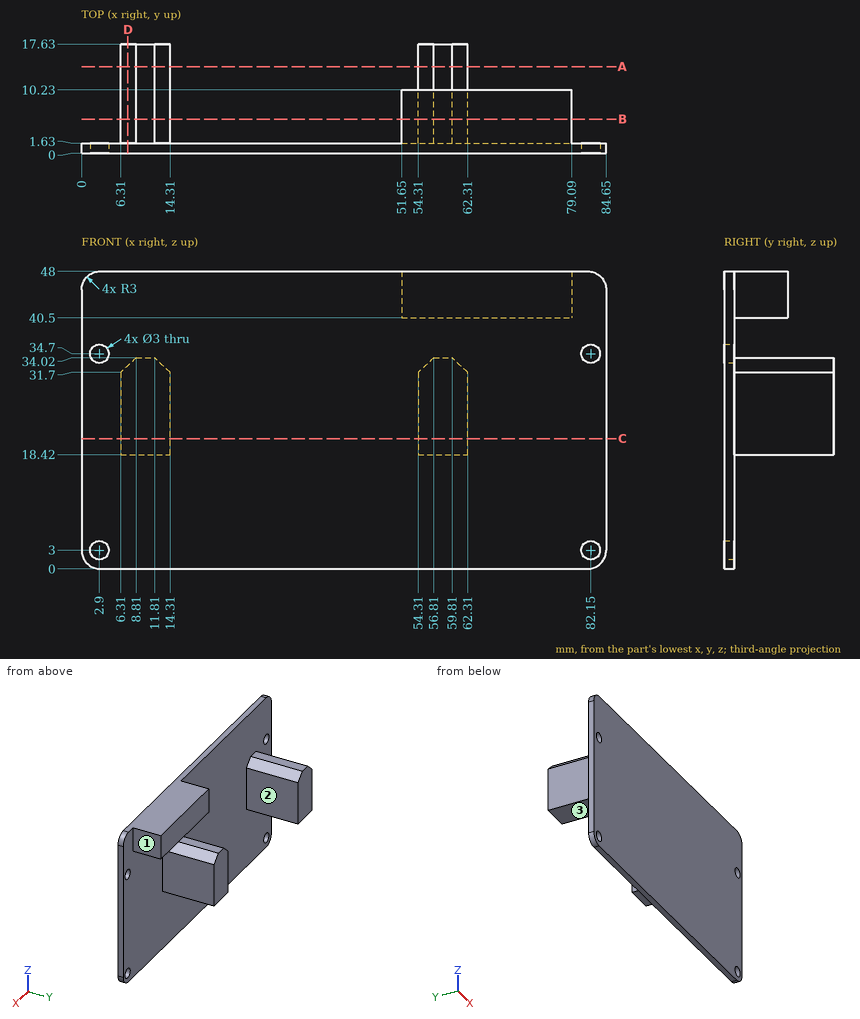
Here's the drawing with two shaded views (mm, measured from the low corner). I have some questions. A direction names the side the tool comes from. Give positions to 0.01 mm unless a question says otherwise; leave off trailing zeros. Loops run counter-clockwise (first coordinate to the right, second up) from the corner with the lowest first, then second, coordinate; pieces in that order, holes last. Notation, with made-up numbers: (-27, 18) -> (22, 18) arc R11 ccw to (22, 25) -> close; hole circle Ø5 at (0, -14). An arc over 180 degrees is marked (long way). Use one line per item in the form item = value.
1) If we section it at B-B (y = 5.5): Please give me the cut outline in (x, z), plus the area to 3 significant figures.
Answers:
outline = (6.31, 18.42) -> (14.31, 18.42) -> (14.31, 31.7) -> (11.81, 34.02) -> (8.81, 34.02) -> (6.31, 31.7) -> close; (51.65, 40.5) -> (79.09, 40.5) -> (79.09, 48) -> (51.65, 48) -> close; (54.31, 18.42) -> (62.31, 18.42) -> (62.31, 31.7) -> (59.81, 34.02) -> (56.81, 34.02) -> (54.31, 31.7) -> close
area = 444 mm²
2) I need wall thicknesses on line 1 along X through (y, z) = (1.3, 3); line 2 along Y through (x, z) = (15.5, 7); line 3 along Z through (x, y) = (11, 5.75). Which ranges of each line are inside material? Lowest first, please.
Answers:
line_1 = 0 to 1.4, 4.4 to 80.65, 83.65 to 84.65
line_2 = 0 to 1.63
line_3 = 18.42 to 34.02
3) If we section it at A-A (y = 14): Please give me the cut outline in (x, z).
Answers:
outline = (6.31, 18.42) -> (14.31, 18.42) -> (14.31, 31.7) -> (11.81, 34.02) -> (8.81, 34.02) -> (6.31, 31.7) -> close; (54.31, 18.42) -> (62.31, 18.42) -> (62.31, 31.7) -> (59.81, 34.02) -> (56.81, 34.02) -> (54.31, 31.7) -> close
4) For the marked faces 1, 2 and 3, which set-ups out of +Z, -Z, +X, -X, +Y, -Y let a thin tool reach every point of the face, with its end or its side?
Answers:
face_1 = +Z, -Z, +X, +Y
face_2 = +Z, -Z, +Y
face_3 = -Z, +X, -X, +Y
5) Will these pins go through, and if not, where does the flat tip stop? pin 1 (4 mm diameter, centred on x = 9, y = 11.5, fed in from -Z); pin 2 (9.5 mm diameter, centred on x = 68.5, y = 7.5, fed in from -Z); pin 3 (3 mm diameter, centred on x = 49.5, z = 12.5, fed in from +Y).
Answers:
pin_1 = 18.42
pin_2 = 40.5
pin_3 = 1.63
6) If we section it at D-D (x = 7.5): Please give me the cut outline in (y, z), plus the area to 3 significant figures.
Answers:
outline = (0, 0) -> (1.63, 0) -> (1.63, 18.42) -> (17.63, 18.42) -> (17.63, 32.8) -> (1.63, 32.8) -> (1.63, 48) -> (0, 48) -> close
area = 308 mm²
7) If we section it at C-C (z = 21): Please give me the cut outline in (x, y), plus the area to 3 significant figures.
Answers:
outline = (0, 0) -> (84.65, 0) -> (84.65, 1.63) -> (62.31, 1.63) -> (62.31, 17.63) -> (54.31, 17.63) -> (54.31, 1.63) -> (14.31, 1.63) -> (14.31, 17.63) -> (6.31, 17.63) -> (6.31, 1.63) -> (0, 1.63) -> close
area = 394 mm²
